Check sheet for the modelled part. Datum: model origin and axes. Units: mm. Face numbers are marked on the shaded views. A direction names the side the tool comes from. Coordinates: 2 decimals unless noted, no trailing zeros. Write each loop counter-clockwise with the first axis right and the second up, starting at its lowest first coordinate (ties: lowest second). Pieces come first, ordered by that corner, then holes. Notation, with made-up numbers: (-22.75, 54) -> (17.25, 54) arc R27 cw to (17.25, 87) -> close; hole circle Ø8 at (58.25, -4). An arc over 180 degrees is marked (long way). One line per item, written item: value. Start each with the question number.
1) Sectioned sample at C-C on x = 9.5. Enter the section's corners in (y, z).
2) Set-up check for the marked faces 1, 2 and 3: record each of +Z, -Z, +X, -X, +Y, -Y from which the full face is reachable in a straight line by a thin tool's end or side.
3) Sectioned sample at A-A on z = 0. Enter the section's corners in (x, y).
4) Gauge pin test, flat ends, axial feed: P1, Ø3, axis at y = 1.5, z = 5.5, coming from the +X side; P2, Ø1.5, axis at x = 3.5, y = 5, coming from the +Z side; P3, Ø4, axis at x = -4.5, y = 2, coming from the -Z side. Record the tip position at first contact, or that the pin passes through.
5) Sectioned sample at B-B on z = -4.5. Enter the section's corners in (x, y).
6) Draft check along X on the marked faces 4, 5 and 6. Enter one of: +X half, -X half, draft (parallel to the pull), parting line (faces both ways), or undercut.
7) Sectioned sample at D-D on x = 3.5. Enter the section's corners in (y, z), plus the area to 3 significant figures.
8) Scan lines: line 1 along X through (y, z) = (5.5, 0); line 2 along X through (y, z) = (4, -8); line 3 along Z through (x, y) = (-6.75, 3.25). Record each from-to range of solid material in increasing order. Write a range as [from, to].
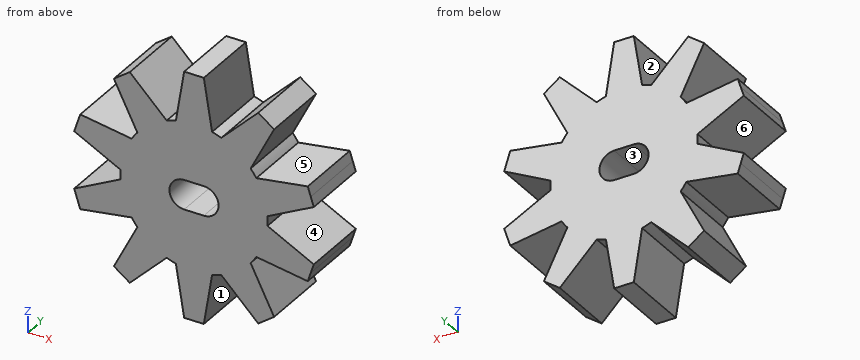
Autodesk Inventor part; units mm, degrees
sketch "Sketch1" plane through (0, 0, 0) normal (0, 1, 0) x (-1, 0, 0)
  circle A0 centre (0, 0) radius 7.5
  dimension "d0" = 15
extrude "Extrusion1" add sketch "Sketch1" along normal blind 7
sketch "Sketch2" plane through (0, 7, 0) normal (0, 1, 0) x (1, 0, 0)
  line L0 (0, 0) -> (2.5, 0)
  line L1 (2.5, 0) -> (-2.5, 0) construction
  line L2 (1, 1.5) -> (-1, 1.5)
  line L3 (-1, -1.5) -> (1, -1.5)
  arc A0 (1, -1.5) -> (1, 1.5) centre (1, 0) ccw
  arc A1 (-1, 1.5) -> (-1, -1.5) centre (-1, 0) ccw
  dimension "d3" = 2.5
  dimension "d4" = 5
  dimension "d5" = 3
extrude "Extrusion2" cut sketch "Sketch2" against normal blind 7
sketch "Sketch3" plane through (0, 0, 0) normal (0, 1, 0) x (-1, 0, 0)
  circle A0 centre (0, 0) radius 7.5
  line L0 (0, 12.5) -> (1, 12.5)
  line L1 (1, 12.5) -> (1.844, 7.2698)
  line L2 (-1, 12.5) -> (-1.844, 7.2698)
  line L3 (0, 12.5) -> (-1, 12.5)
  line L4 (-7.3473, 10.1127) -> (-6.5383, 10.7005)
  line L5 (-7.3473, 10.1127) -> (-8.1563, 9.5249)
  line L6 (-8.1563, 9.5249) -> (-5.7649, 4.7975)
  line L7 (-6.5383, 10.7005) -> (-2.7813, 6.9652)
  line L8 (-11.8882, 3.8627) -> (-11.5792, 4.8138)
  line L9 (-11.8882, 3.8627) -> (-12.1972, 2.9117)
  line L10 (-12.1972, 2.9117) -> (-7.4838, 0.4928)
  line L11 (-11.5792, 4.8138) -> (-6.3442, 4.0002)
  line L12 (-11.8882, -3.8627) -> (-12.1972, -2.9117)
  line L13 (-11.8882, -3.8627) -> (-11.5792, -4.8138)
  line L14 (-11.5792, -4.8138) -> (-6.3442, -4.0002)
  line L15 (-12.1972, -2.9117) -> (-7.4838, -0.4928)
  line L16 (-7.3473, -10.1127) -> (-8.1563, -9.5249)
  line L17 (-7.3473, -10.1127) -> (-6.5383, -10.7005)
  line L18 (-6.5383, -10.7005) -> (-2.7813, -6.9652)
  line L19 (-8.1563, -9.5249) -> (-5.7649, -4.7975)
  line L20 (0, -12.5) -> (-1, -12.5)
  line L21 (0, -12.5) -> (1, -12.5)
  line L22 (1, -12.5) -> (1.844, -7.2698)
  line L23 (-1, -12.5) -> (-1.844, -7.2698)
  line L24 (7.3473, -10.1127) -> (6.5383, -10.7005)
  line L25 (7.3473, -10.1127) -> (8.1563, -9.5249)
  line L26 (8.1563, -9.5249) -> (5.7649, -4.7975)
  line L27 (6.5383, -10.7005) -> (2.7813, -6.9652)
  line L28 (11.8882, -3.8627) -> (11.5792, -4.8138)
  line L29 (11.8882, -3.8627) -> (12.1972, -2.9117)
  line L30 (12.1972, -2.9117) -> (7.4838, -0.4928)
  line L31 (11.5792, -4.8138) -> (6.3442, -4.0002)
  line L32 (11.8882, 3.8627) -> (12.1972, 2.9117)
  line L33 (11.8882, 3.8627) -> (11.5792, 4.8138)
  line L34 (11.5792, 4.8138) -> (6.3442, 4.0002)
  line L35 (12.1972, 2.9117) -> (7.4838, 0.4928)
  line L36 (7.3473, 10.1127) -> (8.1563, 9.5249)
  line L37 (7.3473, 10.1127) -> (6.5383, 10.7005)
  line L38 (6.5383, 10.7005) -> (2.7813, 6.9652)
  line L39 (8.1563, 9.5249) -> (5.7649, 4.7975)
  dimension "d9" = 1
  dimension "d12" = 360
extrude "Extrusion3" add sketch "Sketch3" along normal blind 7 contours A0 L34 L33 L32 L35 | L30 L29 L28 L31 A0 | A0 L38 L37 L36 L39 | L26 L25 L24 L27 A0 | A0 L2 L3 L0 L1 | L22 L21 L20 L23 A0 | A0 L6 L5 L4 L7 | L18 L17 L16 L19 A0 | A0 L10 L9 L8 L11 | L14 L13 L12 L15 A0
properties part number "zahnrad"
Answers:
1. outline: (0, -4.49) -> (7, -4.49) -> (7, -1.53) -> (0, -1.53) -> close; (0, 1.53) -> (7, 1.53) -> (7, 4.49) -> (0, 4.49) -> close
2. face 1: -Z, +Y, -Y
2. face 2: +Z, +Y, -Y
2. face 3: +Y, -Y
3. outline: (-7.5, 0) -> (-2.5, 0) -> (-2.5, 7) -> (-7.5, 7) -> close; (2.5, 0) -> (7.5, 0) -> (7.5, 7) -> (2.5, 7) -> close
4. P1: stops at x = 11.84
4. P2: stops at z = 8.43
4. P3: stops at z = -10.66
5. outline: (-11.68, 0) -> (-9.56, 0) -> (-9.56, 7) -> (-11.68, 7) -> close; (-6, 0) -> (6, 0) -> (6, 7) -> (-6, 7) -> close; (9.56, 0) -> (11.68, 0) -> (11.68, 7) -> (9.56, 7) -> close
6. face 4: +X half
6. face 5: undercut
6. face 6: -X half
7. outline: (0, -7.68) -> (7, -7.68) -> (7, 7.68) -> (0, 7.68) -> close
7. area: 108 mm2
8. line 1: x = [-7.5, -2.5], [2.5, 7.5]
8. line 2: x = [-7.38, -3.82], [-1.73, 1.73], [3.82, 7.38]
8. line 3: z = [-10.55, -6.74], [-4.06, 4.06], [6.74, 10.55]
